Part model, mm, in its own coordinate system. A direction names the side the tool comes from. Round coordinates to 2 decimals unless told otherwise and drop trailing zeros. Loops run counter-clockwise (first coordinate to the right, second up) from the corner with the lowest first, then second, coordinate; pieces in that order, holes last. Notation, with made-up numbers: (80, 46) -> (96, 46) arc R21 cw to (96, 76) -> close; hole circle Ø1 at (23, -39.5). An arc over 180 degrees is marked (long way). Use a Markdown table: item, result. Add a question column.
Item 1: Cut at A-A, the plane x = 0. List the corners of the cut face in (y, z), plus the area to 3 significant figures.
Item 2: Two-plate mould, pull along X, no slides. Class faces 4 (the face through (-42, 1, 0)), 5 (the face through (-35.15, 2.46, -32.99)), 6 (the face through (-13, 15.5, -1)): pulls with the +X half, pulls with the -X half, needs draft (parallel to the pull), parting line crosses it, or undercut.
Item 3: Probe line 1 (Z direction, x = 32, y = 1.6); line 2 (X direction, y = 1, z = -33); line 3 (X direction, y = 3.6, z = -32). List the from-to ranges inside material, lowest first. Write a range as [from, to].
Item 4: Which spindle directions (+Z, -Z, +X, -X, +Y, -Y) get a long thin tool onto all of the face, cutting with end or side? Do faces 1 (the face through (5, 5, 7)), 2 (the face through (-8.095, 1.981, 5.161)), 3 (the face through (28.95, 2.46, -30.74)). Say none if no direction does.
Item 5: Cut at D-D, the plane y = 13. List the corners of the cut face in (x, z), plus the area to 3 significant figures.
Item 6: Flat gauge pins, fed straight in: pin 1 (5 mm diameter, centred on x = 14, y = 6, fed in from +Z); pin 2 (15.5 mm diameter, centred on x = 0, z = 0, fed in from -Y); pin 3 (4 mm diameter, centred on x = 32, z = -32, fed in from +Y); pin 4 (1 mm diameter, centred on x = -7.5, y = 9.5, fed in from +Z). Where does each tip first touch, or does it go through?
Item 7: Cut at B-B, the plane z = 0. List the corners of the cut face in (x, y).
Item 8: Cut at C-C, the plane x = 26. List the corners of the cut face in (y, z).
```python
from build123d import *

# Parameters (mm, degrees)
BOSS_EXTRUDE1_DEPTH      = 5
FILLET1_R                = 3
M6_CLEARANCE_HOLE1_D     = 6.6
M6_CLEARANCE_HOLE1_DEPTH = 8
M6_CLEARANCE_HOLE1_TIP   = 1.982840043


with BuildPart() as part:
    # Sketch1 → Boss-Extrude1 (new body)
    with BuildSketch(Plane(origin=(0, 0, 0), x_dir=(1, 0, 0), z_dir=(0, 1, 0))):
        with BuildLine():
            Line((32, 42), (-32, 42))
            ThreePointArc((-32, 42), (-39.071067812, 39.071067812), (-42, 32))
            Line((-42, 32), (-42, -32))
            ThreePointArc((-42, -32), (-39.071067812, -39.071067812), (-32, -42))
            Line((-32, -42), (32, -42))
            ThreePointArc((32, -42), (39.071067812, -39.071067812), (42, -32))
            Line((42, -32), (42, 32))
            ThreePointArc((42, 32), (39.071067812, 39.071067812), (32, 42))
        make_face()
    extrude(amount=BOSS_EXTRUDE1_DEPTH)

    # Sketch3 → Revolve2 (revolve)
    with BuildSketch(Plane.XY, mode=Mode.PRIVATE) as revolve2_sk:
        with BuildLine():
            Line((-22.25, 5), (-12.5, 5))
            Line((-12.5, 5), (-11.15, 5))
            Line((-11.15, 5), (-11.15, 14))
            Line((-11.15, 14), (-12.5, 14))
            ThreePointArc((-12.5, 14), (-15.66727432, 7.649963846), (-22.25, 5))
        make_face()
        with BuildLine():
            Line((-12.5, 14), (-11.15, 14))
            ThreePointArc((-11.15, 14), (-11.537197996, 15.009021804), (-12.5, 15.5))
            Line((-12.5, 15.5), (-15.5, 15.5))
            ThreePointArc((-15.5, 15.5), (-13.822949017, 15.104101966), (-12.5, 14))
        make_face()
    revolve(revolve2_sk.sketch.rotate(Axis((0, 0, 0), (0, -1, 0)), 270), axis=Axis((0, 0, 0), (0, -1, 0)))

    # Sketch3_5 → Cut-Revolve2 (revolve, cut)
    with BuildSketch(Plane.XY, mode=Mode.PRIVATE) as cut_revolve2_sk:
        with BuildLine():
            Line((0, 0), (0, 5))
            Line((0, 5), (-7.6, 5))
            ThreePointArc((-7.6, 5), (-8.694616444, 4.701278719), (-9.6, 4.017392631))
            Line((-9.6, 4.017392631), (-9.6, 0))
            Line((-9.6, 0), (0, 0))
        make_face()
    revolve(cut_revolve2_sk.sketch.rotate(Axis((0, 0, 0), (0, -1, 0)), 270), axis=Axis((0, 0, 0), (0, -1, 0)), mode=Mode.SUBTRACT)

    # Fillet1
    fillet1_edges = [part.edges().sort_by_distance(p)[0] for p in [
        (39.071067812, 5, 39.071067812),
        (0, 5, 42),
        (-39.071067812, 5, 39.071067812),
        (-42, 5, 0),
        (-39.071067812, 5, -39.071067812),
        (0, 5, -42),
        (39.071067812, 5, -39.071067812),
        (42, 5, 0),
    ]]
    fillet(fillet1_edges, radius=FILLET1_R)

    # M6 Clearance Hole1
    with Locations(Plane(origin=(0, 5, 0), x_dir=(1, 0, 0), z_dir=(0, 1, 0))):
        with Locations((-32, 32), (-32, -32), (32, -32), (32, 32)):
            Hole(M6_CLEARANCE_HOLE1_D / 2, depth=M6_CLEARANCE_HOLE1_DEPTH)
            with Locations((0, 0, -(M6_CLEARANCE_HOLE1_DEPTH + M6_CLEARANCE_HOLE1_TIP / 2))):  # 118° drill point
                Cone(0, M6_CLEARANCE_HOLE1_D / 2, M6_CLEARANCE_HOLE1_TIP, mode=Mode.SUBTRACT)


solid = part.part
```
A:
| question | item | result |
|---|---|---|
| 1 | outline | (0, -42) -> (2, -42) arc R3 ccw to (5, -39) -> (5, -22.25) arc R10 cw to (14, -12.5) arc R3.75 cw to (15.5, -15.5) -> (15.5, -12.5) arc R1.51 ccw to (14, -11.15) -> (5, -11.15) -> (5, -7.6) arc R3 cw to (4.02, -9.6) -> (0, -9.6) -> close; (0, 9.6) -> (4.02, 9.6) arc R3 cw to (5, 7.6) -> (5, 11.15) -> (14, 11.15) arc R1.51 ccw to (15.5, 12.5) -> (15.5, 15.5) arc R3.75 cw to (14, 12.5) arc R10 cw to (5, 22.25) -> (5, 39) arc R3 ccw to (2, 42) -> (0, 42) -> close |
| 1 | area | 394 mm^2 |
| 2 | face 4 | pulls with the -X half |
| 2 | face 5 | undercut |
| 2 | face 6 | needs draft |
| 3 | line 1 | z = [-42, -35.3], [-28.7, 28.7], [35.3, 42] |
| 3 | line 2 | x = [-41.95, -35.14], [-28.86, 28.86], [35.14, 41.95] |
| 3 | line 3 | x = [-41.54, -35.3], [-28.7, 28.7], [35.3, 41.54] |
| 4 | face 1 | +Y |
| 4 | face 2 | -Y |
| 4 | face 3 | +Y, -Y |
| 5 | outline | circle Ø25.3 at (0, 0); hole circle Ø22.3 at (0, 0) |
| 5 | area | 112 mm^2 |
| 6 | pin 1 | stops at z = 41.6 |
| 6 | pin 2 | stops at y = 4.98 |
| 6 | pin 3 | passes through |
| 6 | pin 4 | stops at z = 12.44 |
| 7 | outline | (-42, 0) -> (-9.6, 0) -> (-9.6, 4.02) arc R3 cw to (-7.6, 5) -> (-11.15, 5) -> (-11.15, 14) arc R1.51 ccw to (-12.5, 15.5) -> (-15.5, 15.5) arc R3.75 cw to (-12.5, 14) arc R10 cw to (-22.25, 5) -> (-39, 5) arc R3 ccw to (-42, 2) -> close; (7.6, 5) arc R3 cw to (9.6, 4.02) -> (9.6, 0) -> (42, 0) -> (42, 2) arc R3 ccw to (39, 5) -> (22.25, 5) arc R10 cw to (12.5, 14) arc R3.75 cw to (15.5, 15.5) -> (12.5, 15.5) arc R1.51 ccw to (11.15, 14) -> (11.15, 5) -> close |
| 8 | outline | (0, -42) -> (2, -42) arc R3 ccw to (5, -39) -> (5, 39) arc R3 ccw to (2, 42) -> (0, 42) -> close |
